```python
from build123d import *

# Parameters (mm, degrees)
SCHIZZO1_W                   = 69.56
SCHIZZO1_H                   = 10
ESTRUSIONE_ESTRUSIONE1_DEPTH = 5
SCHIZZO2_R                   = 4.15
ESTRUSIONE_ESTRUSIONE2_DEPTH = 10
SCHIZZO3_R                   = 1.65
TAGLIO_ESTRUSIONE1_DEPTH     = 5


with BuildPart() as part:
    # Schizzo1 → Estrusione-Estrusione1 (new body)
    with BuildSketch(Plane.XY):
        Rectangle(SCHIZZO1_W, SCHIZZO1_H)
    extrude(amount=ESTRUSIONE_ESTRUSIONE1_DEPTH)

    # Schizzo2 → Estrusione-Estrusione2 (add)
    with BuildSketch(Plane.XZ.offset(5)):
        with BuildLine():
            Line((24.621255453, 0), (-24.621255453, 0))
            Line((-24.621255453, 0), (-6.857549921, -15.584245975))
            ThreePointArc((-6.857549921, -15.584245975), (0, -17.026294768), (6.857549921, -15.584245975))
            Line((6.857549921, -15.584245975), (24.621255453, 0))
        make_face()
        with Locations(Location((0, -10.460161878, 0), (0, 0, 270))):
            Circle(SCHIZZO2_R, mode=Mode.SUBTRACT)
    extrude(amount=-ESTRUSIONE_ESTRUSIONE2_DEPTH)

    # Schizzo3 → Taglio-Estrusione1 (cut)
    with BuildSketch(Plane(origin=(0, 0, 0), x_dir=(-1, 0, 0), z_dir=(0, 0, -1))):
        with Locations((-29.700627727, 0)):
            Circle(SCHIZZO3_R)
    taglio_estrusione1 = extrude(amount=-TAGLIO_ESTRUSIONE1_DEPTH, mode=Mode.SUBTRACT)

    # Specchia1: Taglio-Estrusione1 across plane
    add(taglio_estrusione1.mirror(Plane(origin=(0, 0, 0), x_dir=(0, 0, 1), z_dir=(1, 0, 0))), mode=Mode.SUBTRACT)


solid = part.part
```
CAD build for the part. Positions are in the model's coordinates, mm. A direction names the side the tool comes from. Coordinates: 2 decimals unless noted, no trailing zeros. Order: outer loops, then holes, each group sorted by start corner. A loop starts at its lowest first (then second) coordinate and runs counter-clockwise, first axis right, second up. Notation, with made-up numbers: (81, -14.5) -> (93, -14.5) arc R30 ccw to (93, 18.5) -> close; hole circle Ø3 at (28, 27). An arc over 180 degrees is marked (long way). Use one line per item in the form item = value. Start each with the question number.
1) Drop flat-ended pins along their axis: pin 1 (5.5 mm diameter, centred on x = 29.7, y = 0, fed in from -Z); pin 2 (5 mm diameter, centred on x = -20, z = -10, fed in from -Y); pin 3 (2 mm diameter, centred on x = -4, y = -1.5, fed in from -Z). Give the stop position or say it passes through.
2) Drill centre lines: L1, parallel to Z at x = -26, y = -1.75; L2, parallel to X at y = -3, z = -13; L3, parallel to X at y = 3.5, z = -10. Where is each one in solid material? Low to high. Write a range as [from, to].
3) Band-saw the part on D-D on z = 2.75. Give the cut face in (x, y).
4) Band-saw the part on B-B on x = 0. Give the cut face in (y, z), then the cut area to 3 significant figures.
5) Tool access for faces 4 (the cylindrical face through (-2.53, -0.07, -7.17)), 5 (the flat face through (30, 2, 0)): list every direction of +Z, -Z, +X, -X, +Y, -Y with a clear straight run to the whole face (end or side of a thin tool).
6) Pull direction Y, two halves, no side cores. Call faces 1 (the flat face through (0, -5, -1)), 2 (the cylindrical face through (-31.35, 0.07, 2.46)), 3 (the flat face through (-30, 2, 0)): +Y half, -Y half, draft (parallel to the pull), parting line (faces both ways), or undercut.
7) Band-saw the part on C-C on y = 3.5. Give the cut face in (x, z), then the cut area to 3 significant figures.
8) Band-saw the part on A-A on y = 0. Give the cut face in (x, z), then the cut area to 3 significant figures.
Entries:
q1.pin_1 = 0
q1.pin_2 = through
q1.pin_3 = -16.76
q2.L1 = [0, 5]
q2.L2 = [-9.8, -3.28], [3.28, 9.8]
q2.L3 = [-13.22, -4.12], [4.12, 13.22]
q3.outline = (-34.78, -5) -> (34.78, -5) -> (34.78, 5) -> (-34.78, 5) -> close; hole circle Ø3.3 at (-29.7, 0); hole circle Ø3.3 at (29.7, 0)
q4.outline = (-5, -17.03) -> (5, -17.03) -> (5, -14.61) -> (-5, -14.61) -> close; (-5, -6.31) -> (5, -6.31) -> (5, 5) -> (-5, 5) -> close
q4.area = 137 mm2
q5.face_4 = +Y, -Y
q5.face_5 = -Z, +X, +Y, -Y
q6.face_1 = -Y half
q6.face_2 = undercut
q6.face_3 = draft
q7.outline = (-34.78, 0) -> (-24.62, 0) -> (-6.86, -15.58) arc R17.03 ccw to (6.86, -15.58) -> (24.62, 0) -> (34.78, 0) -> (34.78, 5) -> (-34.78, 5) -> close; hole circle Ø8.3 at (0, -10.46)
q7.area = 798 mm2
q8.outline = (-34.78, 0) -> (-31.35, 0) -> (-31.35, 5) -> (-34.78, 5) -> close; (-28.05, 0) -> (-24.62, 0) -> (-6.86, -15.58) arc R17.03 ccw to (6.86, -15.58) -> (24.62, 0) -> (28.05, 0) -> (28.05, 5) -> (-28.05, 5) -> close; (31.35, 0) -> (34.78, 0) -> (34.78, 5) -> (31.35, 5) -> close; hole circle Ø8.3 at (0, -10.46)
q8.area = 765 mm2
